Geometry: final body of the model. Coordinates: model frame, mm. Face numbers are marked on the shaded views. A direction names the side the tool comes from. Coordinates: 2 decimals unless noted, no trailing zeros. Write each loop counter-clockwise with the first axis right and the second up, starting at its lowest first coordinate (ties: lowest second). Pieces come first, ordered by that corner, then holes. Notation, with made-up numbers: (-36.75, -22) -> (20.25, -22) arc R13 cw to (20.25, -9) -> close; hole circle Ø1 at (5, 36.5). An arc over 180 degrees is marked (long way). Answer as a JSON object with one key per item and string values. Group by question number.
```python
from build123d import *

# Parameters (mm, degrees)
SKETCH1_W           = 53.7972
SKETCH1_H           = 23.876
BOSS_EXTRUDE1_DEPTH = 1.4478
SKETCH2_R           = 1.68275
CUT_EXTRUDE1_DEPTH  = 30.464328446
SKETCH3_R           = 5.08
BOSS_EXTRUDE2_DEPTH = 10.16
SKETCH4_W           = 11.43
SKETCH4_H           = 15.875
BOSS_EXTRUDE3_DEPTH = 9.144
SKETCH5_W           = 9.4742
SKETCH5_H           = 4.2164
BOSS_EXTRUDE4_DEPTH = 9.144
SKETCH6_R           = 1.1176
BOSS_EXTRUDE5_DEPTH = 1.524
SKETCH7_W           = 15.875
SKETCH7_H           = 8.128
BOSS_EXTRUDE6_DEPTH = 16.0528


with BuildPart() as part:
    # Sketch1 → Boss-Extrude1 (new body)
    with BuildSketch(Plane(origin=(0, 0, 0), x_dir=(1, 0, 0), z_dir=(0, 1, 0))):
        Rectangle(SKETCH1_W, SKETCH1_H)
    extrude(amount=BOSS_EXTRUDE1_DEPTH)

    # Sketch2 → Cut-Extrude1 (cut, through all)
    with BuildSketch(Plane(origin=(0, 1.4478, 0), x_dir=(1, 0, 0), z_dir=(0, 1, 0))):
        with Locations(Location((17.5768, -9.29005, 0), (0, 0, 270))):
            Circle(SKETCH2_R)
        with Locations(Location((-17.5768, 9.29005, 0), (0, 0, 270))):
            Circle(SKETCH2_R)
    extrude(amount=-CUT_EXTRUDE1_DEPTH, mode=Mode.SUBTRACT)

    # Sketch3 → Boss-Extrude2 (add)
    with BuildSketch(Plane(origin=(0, 1.4478, 0), x_dir=(1, 0, 0), z_dir=(0, 1, 0))):
        with Locations(Location((20.5486, 0, 0), (0, 0, 270))):
            Circle(SKETCH3_R)
        with Locations(Location((-20.5486, 0, 0), (0, 0, 270))):
            Circle(SKETCH3_R)
    extrude(amount=BOSS_EXTRUDE2_DEPTH)

    # Sketch4 → Boss-Extrude3 (add)
    with BuildSketch(Plane(origin=(0, 1.4478, 0), x_dir=(1, 0, 0), z_dir=(0, 1, 0))):
        with Locations((-8.4836, -4.0005)):
            Rectangle(SKETCH4_W, SKETCH4_H)
    extrude(amount=BOSS_EXTRUDE3_DEPTH)

    # Sketch5 → Boss-Extrude4 (add)
    with BuildSketch(Plane(origin=(0, 1.4478, 0), x_dir=(1, 0, 0), z_dir=(0, 1, 0))):
        with Locations((-3.8735, 9.8298)):
            Rectangle(SKETCH5_W, SKETCH5_H)
    extrude(amount=BOSS_EXTRUDE4_DEPTH)

    # Sketch6 → Boss-Extrude5 (add)
    with BuildSketch(Plane(origin=(0, 10.5918, 0), x_dir=(1, 0, 0), z_dir=(0, 1, 0))):
        with Locations(Location((-7.3406, 10.668, 0), (0, 0, 90))):
            Circle(SKETCH6_R)
    extrude(amount=BOSS_EXTRUDE5_DEPTH)

    # Sketch7 → Boss-Extrude6 (add)
    with BuildSketch(Plane(origin=(0, 1.4478, 0), x_dir=(1, 0, 0), z_dir=(0, 1, 0))):
        with Locations((5.1689, 1.016)):
            Rectangle(SKETCH7_W, SKETCH7_H)
    extrude(amount=BOSS_EXTRUDE6_DEPTH)


solid = part.part
```
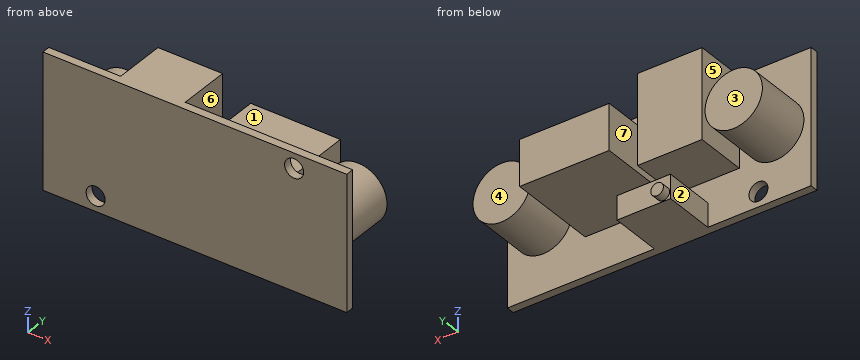
Item 1: Section C-C on y = 2. Output: boundary loops of the cut face in (x, z).
Item 2: Section B-B on z = 0. Output: boundary loops of the cut face in (x, y).
Item 3: Section A-A on x = -3.5. Output: boundary loops of the cut face in (y, z).
Item 4: Section D-D on y = 14.25. Output: boundary loops of the cut face in (x, z), then the cut area to 3 significant figures.
Item 5: Ray query, L1, parallel to X at y = 10.5, z = -2.25; L2, parallel to X at y = 7.25, z = -8.25; L3, parallel to Y at x = 9.5, z = 10. Return the intervals inside material, ascending. Write a range as [from, to].
Item 6: Set-up query: the marked faces 4, 5, 6 and 7. Return all of +Z, -Z, +X, -X, +Y, -Y with unobstructed straight access to the full face (end or side cutting, diameter ignored); none if empty.
Item 7: Mould query, pull axis X, two halves, no side actions, for the marked faces 1, 2 and 3. Classes: +X half, -X half, draft (parallel to the pull), parting line (faces both ways), or undercut.
Item 8: Contact query for flat-ended pins moving along their axis: pin 1 (9 mm diameter, centred on y = 9, z = -3, fed in from -X); pin 2 (6 mm diameter, centred on x = -3, y = 15.5, fed in from +Z); pin 3 (10 mm diameter, centred on x = 11, y = 10.5, fed in from -Z). Output: stop coordinate, or through.
Answer sheet:
{
 "1": {"outline": "circle Ø10.16 at (-20.55, 0); (-14.2, -3.94) -> (-2.77, -3.94) -> (-2.77, -5.08) -> (13.11, -5.08) -> (13.11, 3.05) -> (-2.77, 3.05) -> (-2.77, 11.94) -> (-14.2, 11.94) -> close; (-8.61, -11.94) -> (0.86, -11.94) -> (0.86, -7.72) -> (-8.61, -7.72) -> close; circle Ø10.16 at (20.55, 0)"},
 "2": {"outline": "(-26.9, 0) -> (26.9, 0) -> (26.9, 1.45) -> (25.63, 1.45) -> (25.63, 11.61) -> (15.47, 11.61) -> (15.47, 1.45) -> (13.11, 1.45) -> (13.11, 17.5) -> (-2.77, 17.5) -> (-2.77, 10.59) -> (-14.2, 10.59) -> (-14.2, 1.45) -> (-15.47, 1.45) -> (-15.47, 11.61) -> (-25.63, 11.61) -> (-25.63, 1.45) -> (-26.9, 1.45) -> close"},
 "3": {"outline": "(0, -11.94) -> (10.59, -11.94) -> (10.59, -7.72) -> (1.45, -7.72) -> (1.45, -3.94) -> (10.59, -3.94) -> (10.59, 11.94) -> (0, 11.94) -> close"},
 "4": {"outline": "(-2.77, -5.08) -> (13.11, -5.08) -> (13.11, 3.05) -> (-2.77, 3.05) -> close", "area": "129 mm^2"},
 "5": {"L1": "x = [-25.1, -15.99], [-14.2, 13.11], [15.99, 25.1]", "L2": "x = [-8.61, 0.86]", "L3": "y = [0, 1.45]"},
 "6": {"face 4": "+Z, -Z, +X, +Y", "face 5": "+Z, -Z, +Y", "face 6": "+Z, +Y", "face 7": "+Y"},
 "7": {"face 1": "undercut", "face 2": "-X half", "face 3": "draft"},
 "8": {"pin 1": "stops at x = -25.63", "pin 2": "stops at z = 3.05", "pin 3": "stops at z = -5.08"}
}
